Verification items for the finished model (mm, model axes). Round coordinates to 2 decimals unless told otherwise and drop trailing zeros. Write each loop counter-clockwise with the first axis right and the second up, starting at its lowest first coordinate (ties: lowest second). Pieces come first, ordered by that corner, then holes. Notation, with made-up numbers: (-35, 29) - (9, 29) arc R21 cw to (9, 38) - close; hole circle Ø1 at (-7.5, 82). An arc over 180 degrees is marked (long way). Answer as a JSON object with one key per item and string values. Group by question number.
1) Section check B-B (z = 33.5). Enter the section's corners in (x, y).
2) Section check A-A (x = 42.5). Enter the section's corners in (y, z), then the cut area to 3 significant figures.
3) Go/stop test with a flat-tipped pin: pin 1 Ø1 at (x, y) = (-22, -20.5) entering from -Z. Record where the tip stops, or that it passes through.
4) Thickness scan on line 1 (Y direction, x = 33, z = 35); line 2 (Z direction, x = 35, y = -22.5); line 3 (Y direction, x = -14, z = 37.25). Record the ranges inside material, lowest first.
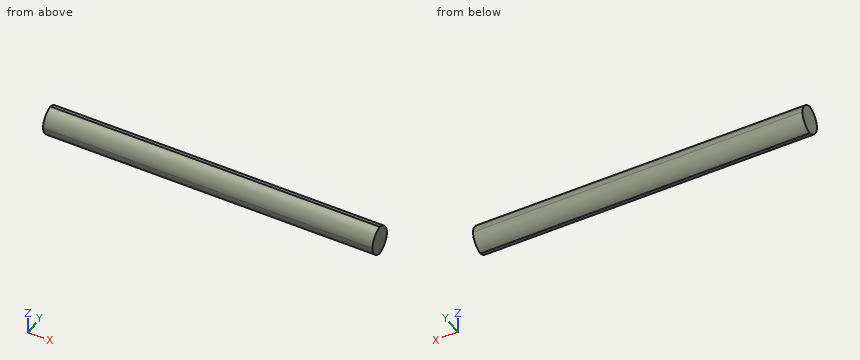
```python
from build123d import *

# Parameters (mm, degrees)
F0_W        = 7.8271683306
F0_H        = 9.5099005848
F2_DEPTH    = 25
F3_DEPTH    = 25
F1_W        = 7.8271683306
F1_H        = 9.5099005848
F4_DEPTH    = 51.5792816877
F3_FACE_W   = 7.8271683306
F3_FACE_H   = 9.5099005848
F4_FACE_W   = 7.8271683306
F4_FACE_H   = 9.5099005848
F6_T1_DEPTH = 126.5792816877


# Not quite as in the source:
# - a fillet or chamfer that OpenCascade refuses, or shapes differently, is made with other operations: its cross-section is extruded or revolved along the edge and cut away or added


with BuildPart() as f2:
    # F0 (on Right) → F2 (new body)
    with BuildSketch(Plane.YZ):
        with Locations((-22.5047236308, 34.8080685362)):
            Rectangle(F0_W, F0_H)
    extrude(amount=F2_DEPTH)

    # F3 (add): a face of the model
    f3_faces = [f2.faces().sort_by_distance(p)[0] for p in [
        (25, -22.5047236308, 34.8080685362),
    ]]
    extrude(f3_faces, amount=F3_DEPTH)

    # F1 (on face) → F4 (join)
    with BuildSketch(Plane.YZ):
        with Locations((-22.5047236308, 34.8080685362)):
            Rectangle(F1_W, F1_H)
    extrude(amount=-F4_DEPTH)

    # F3_face (on face) → F5 section 0
    with BuildSketch(Plane(origin=(50, -22.5047236308, 34.8080685362), x_dir=(0, 1, 0), z_dir=(1, 0, 0))):
        Rectangle(F3_FACE_W, F3_FACE_H)
    # F4_face (on face) → F5 section 1
    with BuildSketch(Plane(origin=(-51.5792816877, -22.5047236308, 34.8080685362), x_dir=(0, 1, 0), z_dir=(-1, 0, 0))):
        Rectangle(F4_FACE_W, F4_FACE_H)
    loft()

    # F6: fillet of radius 5 on 4 edges, made by hand

    # F6_s2 → F6_t1 (cut)
    with BuildSketch(Plane.YZ.offset(-64.0792816877)):
        with BuildLine():
            ThreePointArc((-21.4183077961, 39.5630188286), (-24.9538417021, 38.0985527346), (-26.4183077961, 34.5630188286))
            Line((-26.4183077961, 34.5630188286), (-26.4183077961, 39.5630188286))
            Line((-26.4183077961, 39.5630188286), (-21.4183077961, 39.5630188286))
        make_face()
        with BuildLine():
            ThreePointArc((-23.5911394656, 39.5630188286), (-20.0556055596, 38.0985527346), (-18.5911394656, 34.5630188286))
            Line((-18.5911394656, 34.5630188286), (-18.5911394656, 39.5630188286))
            Line((-18.5911394656, 39.5630188286), (-23.5911394656, 39.5630188286))
        make_face()
        with BuildLine():
            ThreePointArc((-26.4183077961, 35.0531182438), (-24.9538417021, 31.5175843379), (-21.4183077961, 30.0531182438))
            Line((-21.4183077961, 30.0531182438), (-26.4183077961, 30.0531182438))
            Line((-26.4183077961, 30.0531182438), (-26.4183077961, 35.0531182438))
        make_face()
        with BuildLine():
            ThreePointArc((-18.5911394656, 35.0531182438), (-20.0556055596, 31.5175843379), (-23.5911394656, 30.0531182438))
            Line((-23.5911394656, 30.0531182438), (-18.5911394656, 30.0531182438))
            Line((-18.5911394656, 30.0531182438), (-18.5911394656, 35.0531182438))
        make_face()
    extrude(amount=F6_T1_DEPTH, mode=Mode.SUBTRACT)


solid = f2.part
```
Returned:
{
 "1": {"outline": "(-51.58, -26.17) - (50, -26.17) - (50, -18.84) - (-51.58, -18.84) - close"},
 "2": {"outline": "(-26.41, 34.81) arc R5 ccw to (-22.5, 30.17) arc R5 ccw to (-18.6, 34.81) arc R5 ccw to (-22.5, 39.44) arc R5 ccw to start", "area": "53.1 mm2"},
 "3": {"pin 1": "z = 30.78"},
 "4": {"line 1": "-26.4 to -18.61", "line 2": "30.17 to 39.44", "line 3": "-25.63 to -19.37"}
}
